Build history of the part. All positions in model axes, mm. Face numbers are marked on the shaded views. Round coordinates to 2 decimals unless told otherwise and drop trailing zeros. Write each loop counter-clockwise with the first axis right and the second up, starting at its lowest first coordinate (ties: lowest second). Pieces come first, ordered by that corner, then holes.
Item 1: Mould opens along X. For the marked faces 1, 2 and 3 say: +X half, -X half, draft (parallel to the pull), parting line (faces both ways), or undercut.
Item 2: Wall check: probe 1 along Z at (x, y) = (-26, 7); probe 2 along Y at (x, z) = (-1.5, 165); probe 3 along Y at (x, z) = (-27.5, 49.5). Give the ranges that are in metal, low to high.
Item 3: Band-saw the part on B-B, the plane z = 63. Write the cut outline in (x, y), then the cut area to 3 significant figures.
Item 4: Band-saw the part on A-A, the plane x = -24. Write the cut outline in (y, z), then the cut area to 3 significant figures.
Item 5: Band-saw the part on D-D, the plane x = -1.5. Write the cut outline in (y, z).
Item 6: Band-saw the part on C-C, the plane y = -23. Write the cut outline in (x, z), then the cut area to 3 significant figures.
Item 7: Drop flat-ended pins along their axis: pin 1 Ø1.5 at (x, z) = (80, 89) entering from +Y; pin 2 Ø8 at (y, z) = (86, 121) entering from +X; pin 3 Ø17 at (x, y) = (-38.5, 36.5) entering from +Z; pin 4 Ø4 at (x, y) = (-34, -83.5) entering from -Z. Give the stop position or say it passes through.
```python
from build123d import *

# Parameters (mm, degrees)
F1_R     = 111.3933221295
F2_DEPTH = 25.4
F3_R     = 111.3933221295
F3_R_2   = 28.5570056478
F4_DEPTH = 25.4
F5_W     = 62.3087513292
F5_H     = 49.9088813265
F5_R     = 28.5570056478
F6_DEPTH = 127


with BuildPart() as f2:
    # F1 (on face) → F2 (new body)
    with BuildSketch(Plane.XY):
        Circle(F1_R)
    extrude(amount=F2_DEPTH)

    # F3 (on face) → F4 (join)
    with BuildSketch(Plane.XY.offset(25.4)):
        Circle(F3_R)
        with Locations((-24.1107493639, 33.1069529057)):
            Circle(F3_R_2, mode=Mode.SUBTRACT)
    extrude(amount=F4_DEPTH)

    # F5 (on face) → F6 (join)
    with BuildSketch(Plane.XY.offset(50.8)):
        with BuildLine():
            ThreePointArc((111.3933221295, 0), (-98.359674215, 52.2861999324), (62.3087513292, -92.3368383845))
            ThreePointArc((62.3087513292, -92.3368383845), (98.359674215, -52.2861999324), (111.3933221295, 0))
        make_face()
        with Locations((31.1543756646, -67.3823977212)):
            Rectangle(F5_W, F5_H, mode=Mode.SUBTRACT)
        with Locations((-24.1107493639, 33.1069529057)):
            Circle(F5_R, mode=Mode.SUBTRACT)
        with Locations((31.1543756646, -67.3823977212)):
            Rectangle(F5_W, F5_H)
    extrude(amount=F6_DEPTH)


solid = f2.part
```
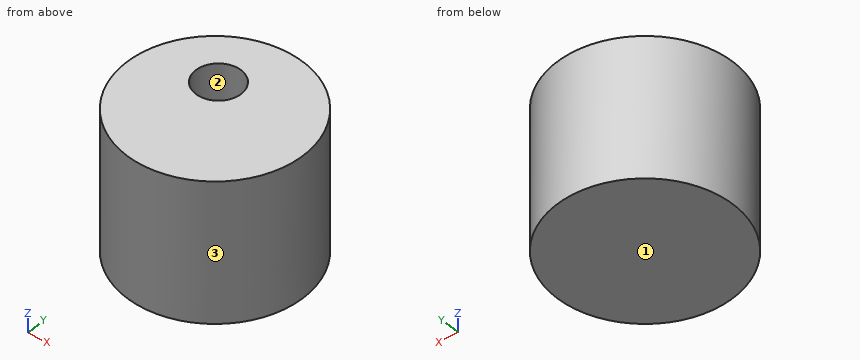
Results:
1. face 1: draft
1. face 2: undercut
1. face 3: parting line
2. probe 1: z = 0 to 25.4
2. probe 2: y = -111.38 to 15.66, 50.55 to 111.38
2. probe 3: y = -107.95 to 4.75, 61.46 to 107.95
3. outline: circle Ø222.79 at (0, 0); hole circle Ø57.11 at (-24.11, 33.11)
3. area: 36,400 mm2
4. outline: (-108.78, 0) - (108.78, 0) - (108.78, 177.8) - (61.66, 177.8) - (61.66, 25.4) - (4.55, 25.4) - (4.55, 177.8) - (-108.78, 177.8) - close
4. area: 30,000 mm2
5. outline: (-111.38, 0) - (111.38, 0) - (111.38, 177.8) - (50.55, 177.8) - (50.55, 25.4) - (15.66, 25.4) - (15.66, 177.8) - (-111.38, 177.8) - close
6. outline: (-108.99, 0) - (108.99, 0) - (108.99, 177.8) - (-108.99, 177.8) - close
6. area: 38,800 mm2
7. pin 1: stops at y = 78.28
7. pin 2: stops at x = 75.4
7. pin 3: stops at z = 25.4
7. pin 4: stops at z = 0
